For this review, take the finished solid that the model builds, in its own axes (mm). A direction names the side the tool comes from. Give positions to 0.01 mm unless a question says otherwise; leave off trailing zeros. Write each loop counter-clockwise with the first axis right and the second up, starting at its lowest first coordinate (ties: lowest second). Pieces come first, ordered by that corner, then holes.
Q1. For line 1 (X direction, y = -5.5, z = -11.5); line 2 (X direction, y = -2.5, z = -2.5); line 3 (X direction, y = 1, z = 3), list the stretches that pass through material, from the lowest coordinate up.
Q2. We need section B-B (x = -11). Write out the cut boundary in (y, z), then the cut area to 3 significant figures.
Q3. Mouldability with a two-part tool opening along Z and no side actions: class faces 1 (the cylindrical face through (-10.11, -3.94, -5.31)), 2 (the flat face through (12.05, 2, -6)), 3 (the flat face through (0, 2, -29)) as released by +Z, released by -Z, zero draft, split by the parting line, or undercut.
Q4. We need section A-A (y = 0.75). Write out the cut boundary in (x, z), then the cut area to 3 significant figures.
Q5. We need section C-C (z = -2.5). Write out the cut boundary in (x, y), then the cut area to 3 significant figures.
Q6. Insertion check: P1, Ø1.8, axis at x = 9, z = -1.5, coming from the +Y side; P2, Ø4, axis at x = 1.5, y = -5.5, coming from the -Z side; P3, Ø1, axis at x = 3.5, y = -5.5, coming from the -Z side (3 decimals). Each pin has a flat end and moves straight along its axis. Give the tip position at first contact, or say it passes through.
Q7. We need section D-D (z = -7). Write out the cut boundary in (x, y), then the cut area to 3 significant figures.
Q8. Machinability: for faces 4 (the flat face through (10.55, -1, 3)), 5 (the flat face through (0, -7, -10)), 6 (the cylindrical face through (0.19, -5.719, -26.594)), which of the approach directions +Z, -Z, +X, -X, +Y, -Y give a long, thin tool a straight path to every point of the face, cutting with its end or side? Answer none if there is none.
```python
from build123d import *

# Parameters (mm, degrees)
SKETCH_R        = 1.65
PAD_DEPTH       = 8
SKETCH001_W     = 12
SKETCH001_H     = 7
POCKET_DEPTH    = 10
POCKET001_DEPTH = 24.101
PAD001_DEPTH    = 24.1
POCKET002_DEPTH = 12
PAD002_DEPTH    = 1.75
POCKET003_DEPTH = 2
PAD003_DEPTH    = 1.5
SKETCH009_W     = 24.1
SKETCH009_H     = 1.5
PAD004_DEPTH    = 1.5
FILLET_R        = 3


with BuildPart() as part:
    # Sketch → Pad (new body)
    with BuildSketch(Plane.XZ):
        Polygon((-12.05, 6), (-12.05, -6), (-12.05, -11), (12.05, -11), (12.05, -6), (12.05, 6), align=None)
        with Locations((-9.75, -3.7)):
            Circle(SKETCH_R, mode=Mode.SUBTRACT)
        with Locations((9.75, -3.7)):
            Circle(SKETCH_R, mode=Mode.SUBTRACT)
    extrude(amount=PAD_DEPTH)

    # Sketch001 (on Face1 of Pad) → Pocket (cut)
    with BuildSketch(Plane(origin=(0, 0, -11), x_dir=(1, 0, 0), z_dir=(0, 0, -1))):
        with Locations((0, 3.5)):
            Rectangle(SKETCH001_W, SKETCH001_H)
    extrude(amount=-POCKET_DEPTH, mode=Mode.SUBTRACT)

    # Sketch003 (on Face8 of Pocket) → Pocket001 (cut, through all)
    with BuildSketch(Plane(origin=(-12.05, 0, 0), x_dir=(0, 0, -1), z_dir=(-1, 0, 0))):
        with BuildLine():
            ThreePointArc((2, 8), (-3.656854, 5.656854), (-6, 0))
            Line((-6, 0), (-6, 8))
            Line((-6, 8), (2, 8))
        make_face()
    extrude(amount=-POCKET001_DEPTH, mode=Mode.SUBTRACT)

    # Sketch004 (on Face8 of Pocket001) → Pad001 (join)
    with BuildSketch(Plane(origin=(-12.05, 0, 0), x_dir=(0, 0, -1), z_dir=(-1, 0, 0))):
        with BuildLine():
            Line((11, 8), (21, 8))
            ThreePointArc((29, 0), (26.656854, 5.656854), (21, 8))
            Line((29, 0), (11, 0))
            Line((11, 0), (11, 8))
        make_face()
    extrude(amount=-PAD001_DEPTH)

    # Sketch005 (on Face4 of Pad001) → Pocket002 (cut)
    with BuildSketch(Plane(origin=(-6, 0, 0), x_dir=(0, 0, 1), z_dir=(1, 0, 0))):
        with BuildLine():
            Line((-11, 7), (-19, 7))
            ThreePointArc((-19, 7), (-23.949747, 4.949747), (-26, 0))
            Line((-26, 0), (-11, 0))
            Line((-11, 0), (-11, 7))
        make_face()
    extrude(amount=POCKET002_DEPTH, mode=Mode.SUBTRACT)

    # Sketch006 (on Face3 of Pocket002) → Pad002 (join)
    with BuildSketch(Plane(origin=(0, 0, 0), x_dir=(1, 0, 0), z_dir=(0, 1, 0))):
        Polygon((-12.05, 6), (-12.05, 29), (12.05, 29), (12.05, 6), (6, 6), (6, 26), (-6, 26), (-6, 6), align=None)
    extrude(amount=PAD002_DEPTH)

    # Sketch007 (on Face2 of Pad002) → Pocket003 (cut)
    with BuildSketch(Plane(origin=(0, 0, 0), x_dir=(1, 0, 0), z_dir=(0, 1, 0))):
        Polygon((-6, 1), (-10.55, 0.999989), (-10.55, -6), (10.55, -6), (10.55, 1), (6, 1), align=None)
    extrude(amount=-POCKET003_DEPTH, mode=Mode.SUBTRACT)

    # Sketch008 (on Face8 of Pocket003) → Pad003 (join)
    with BuildSketch(Plane(origin=(12.05, 0, 0), x_dir=(0, 0, 1), z_dir=(1, 0, 0))):
        with BuildLine():
            Line((-29, 0), (-29, -3.25))
            Line((-29, -3.25), (6, -3.25))
            Line((6, -3.25), (6, 0))
            ThreePointArc((6, 0), (3.656854, 5.656854), (-2, 8))
            Line((-2, 8), (-21, 8))
            ThreePointArc((-21, 8), (-26.656854, 5.656854), (-29, 0))
        make_face()
    pad003 = extrude(amount=PAD003_DEPTH)

    # Mirrored: Pad003 across YZ
    add(pad003.mirror(Plane.YZ))

    # Sketch009 (on Face11 of Mirrored) → Pad004 (join)
    with BuildSketch(Plane(origin=(0, 1.75, 0), x_dir=(1, 0, 0), z_dir=(0, 1, 0))):
        with Locations((0, 28.25)):
            Rectangle(SKETCH009_W, SKETCH009_H)
    extrude(amount=PAD004_DEPTH)

    # Fillet
    fillet_edges = [part.edges().sort_by_distance(p)[0] for p in [
        (-12.05, 2.5, -27.5),
        (12.05, 2.5, -27.5),
    ]]
    fillet(fillet_edges, radius=FILLET_R)


solid = part.part
```
Computed:
1. line 1: x = -13.55 to -6, 6 to 13.55
1. line 2: x = -13.55 to -10.88, -8.62 to -6, 6 to 8.62, 10.88 to 13.55
1. line 3: x = -13.55 to -12.05, 12.05 to 13.55
2. outline: (-8, -21) arc R8 ccw to (0, -29) - (3.25, -29) - (3.25, -26.78) - (1.75, -26.78) - (1.75, -6) - (0, -6) - (0, -4.78) - (-8, -4.78) - close; (-8, -2.62) - (0, -2.62) - (0, 6) arc R8 ccw to (-8, -2) - close
2. area: 279 mm2
3. face 1: undercut
3. face 2: zero draft
3. face 3: released by -Z
4. outline: (-13.55, -29) - (13.55, -29) - (13.55, 6) - (12.05, 6) - (12.05, -6) - (6, -6) - (6, -26) - (-6, -26) - (-6, -6) - (-12.05, -6) - (-12.05, 6) - (-13.55, 6) - close
4. area: 419 mm2
5. outline: (-13.55, -8) - (-10.88, -8) - (-10.88, 0) - (-12.05, 0) - (-12.05, 3.25) - (-13.55, 3.25) - close; (-8.62, -8) - (8.62, -8) - (8.62, 0) - (6, 0) - (6, -7) - (-6, -7) - (-6, 0) - (-8.62, 0) - close; (10.88, -8) - (13.55, -8) - (13.55, 3.25) - (12.05, 3.25) - (12.05, 0) - (10.88, 0) - close
5. area: 106 mm2
6. P1: stops at y = 0
6. P2: stops at z = -28.19
6. P3: stops at z = -27.245
7. outline: (-13.55, -8) - (13.55, -8) - (13.55, 3.25) - (12.05, 3.25) - (12.05, 1.75) - (6, 1.75) - (6, -7) - (-6, -7) - (-6, 1.75) - (-12.05, 1.75) - (-12.05, 3.25) - (-13.55, 3.25) - close
7. area: 164 mm2
8. face 4: +Z, +Y
8. face 5: +Y
8. face 6: -Z, +X, -X, -Y
